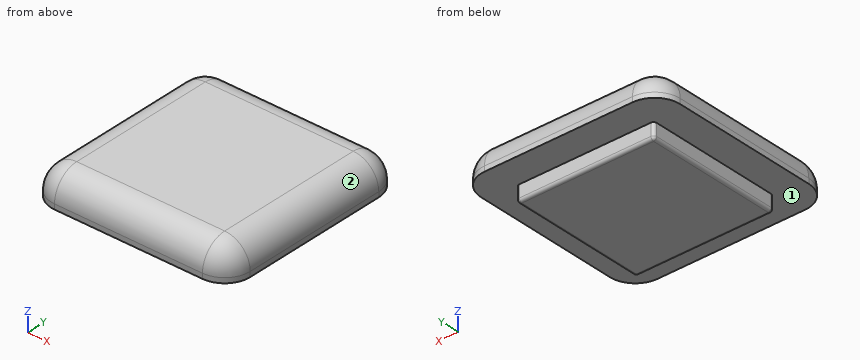
```python
from build123d import *

# Parameters (mm, degrees)
F0_W     = 195
F0_H     = 195
F1_DEPTH = 30
F2_W     = 135
F2_H     = 135
F3_DEPTH = 15
F4_R     = 3
F5_R     = 25
F6_ANGLE = 180


with BuildPart() as f1:
    # F0 (on Top) → F1 (new body)
    with BuildSketch(Plane.XY):
        Rectangle(F0_W, F0_H)
    extrude(amount=F1_DEPTH)

    # F2 (on face) → F3 (join)
    with BuildSketch(Plane.XY.offset(30)):
        Rectangle(F2_W, F2_H)
    extrude(amount=F3_DEPTH)

    # F4
    f4_edges = [f1.edges().sort_by_distance(p)[0] for p in [
        (67.5, 0, 45),
        (0, 67.5, 45),
        (-67.5, 0, 45),
        (0, -67.5, 45),
        (67.5, -67.5, 37.5),
        (67.5, 67.5, 37.5),
        (-67.5, -67.5, 37.5),
        (-67.5, 67.5, 37.5),
    ]]
    fillet(f4_edges, radius=F4_R)

    # F5
    f5_edges = [f1.edges().sort_by_distance(p)[0] for p in [
        (97.5, 0, 0),
        (0, 97.5, 0),
        (-97.5, 0, 0),
        (0, -97.5, 0),
        (97.5, 97.5, 15),
        (-97.5, 97.5, 15),
        (-97.5, -97.5, 15),
        (97.5, -97.5, 15),
    ]]
    fillet(f5_edges, radius=F5_R)


with BuildPart() as f1_1:
    # F6: moved
    add(f1.part.rotate(Axis((97.5, 0, 30), (0, -1, 0)), F6_ANGLE))


with BuildPart() as f1_2:
    # F7: moved
    add(f1_1.part.moved(Location((-195, 0, 0))))


with BuildPart() as f1_3:
    # F8: moved
    add(f1_2.part.moved(Location((0, 0, -15))))


solid = f1_3.part
```
For this review, take the finished solid that the model builds, in its own axes (mm). Face numbers are marked on the shaded views. A direction names the side the tool comes from. Coordinates: 2 decimals unless noted, no trailing zeros. Loops run counter-clockwise (first coordinate to the right, second up) from the corner with the lowest first, then second, coordinate; pieces in that order, holes last. Notation, with made-up numbers: (-27.75, -14.75) -> (11.25, -14.75) arc R14 ccw to (11.25, -8.75) -> close; hole circle Ø5 at (38.5, 8.25). An arc over 180 degrees is marked (long way). Return JSON: item names as keys, results as strings. Group by question number.
(1) Consider section B-B, the plane y = 21. Give the boundary of the cut face in (x, z), plus the area to 3 significant figures.
(2) Consider section A-A, the plane z = 11.5. Give the boundary of the cut face in (x, y), plus the area to 3 significant figures.
(3) Consider section D-D, the plane z = 27. Give the boundary of the cut face in (x, y), plus the area to 3 significant figures.
(4) Tool access review of the marked faces 1 and 2: name each direction out of +Z, -Z, +X, -X, +Y, -Y from which nothing blocks a thin tool from reaching the whole face with its end or side.
(5) For pin 1 Ø1.5 at (y, z) = (69.5, 34.5) entering from +X; pin 2 Ø10 at (y, z) = (62.5, 6) entering from +X; pin 3 Ø6 at (x, z) = (-66.5, 36.5) entering from -Y, all flat-tipped, find the tip position at first contact; note any pin that passes through.
(6) To check wall thickness, follow L1, parallel to X at y = -63.5, z = 10; L2, parallel to Z at x = 65, y = 34. State the ranges of each line that lie inside material, in increasing order.
Results below:
{
 "1": {"outline": "(-97.5, 15) -> (-67.5, 15) -> (-67.5, 3) arc R3 ccw to (-64.5, 0) -> (64.5, 0) arc R3 ccw to (67.5, 3) -> (67.5, 15) -> (97.5, 15) -> (97.5, 20) arc R25 ccw to (72.5, 45) -> (-72.5, 45) arc R25 ccw to (-97.5, 20) -> close", "area": "7,600 mm2"},
 "2": {"outline": "(-67.5, -64.5) arc R3 ccw to (-64.5, -67.5) -> (64.5, -67.5) arc R3 ccw to (67.5, -64.5) -> (67.5, 64.5) arc R3 ccw to (64.5, 67.5) -> (-64.5, 67.5) arc R3 ccw to (-67.5, 64.5) -> close", "area": "18,200 mm2"},
 "3": {"outline": "(-96.5, -72.5) arc R24 ccw to (-72.5, -96.5) -> (72.5, -96.5) arc R24 ccw to (96.5, -72.5) -> (96.5, 72.5) arc R24 ccw to (72.5, 96.5) -> (-72.5, 96.5) arc R24 ccw to (-96.5, 72.5) -> close", "area": "36,800 mm2"},
 "4": {"face 1": "-Z", "face 2": "+Z, +X, +Y, -Y"},
 "5": {"pin 1": "stops at x = 93.38", "pin 2": "stops at x = 67.5", "pin 3": "stops at y = -93.54"},
 "6": {"L1": "x = -67.5 to 67.5", "L2": "z = 0.04 to 45"}
}
